```python
from build123d import *

# Parameters (mm, degrees)
CUT_EXTRUDE_1_DEPTH = 2


with BuildPart() as part:
    # 草图1 → 旋转1 (revolve)
    with BuildSketch(Plane.XY):
        with BuildLine():
            Line((0, 10.8), (-2.4, 10.8))
            ThreePointArc((-2.4, 10.8), (-2.682842712, 10.682842712), (-2.8, 10.4))
            Line((-2.8, 10.4), (-2.8, 8.4))
            ThreePointArc((-2.8, 8.4), (-2.682842712, 8.117157288), (-2.4, 8))
            Line((-2.4, 8), (-1.2, 8))
            Line((-1.2, 8), (-1.2, 7))
            Line((-1.2, 7), (-1.5, 7))
            Line((-1.5, 7), (-1.5, 0))
            Line((-1.5, 0), (0, 0))
            Line((0, 0), (0, 10.8))
        make_face()
    revolve(axis=Axis((0, 0, 0), (0, 1, 0)))

    # 草图2 → 切除-拉伸1 (cut)
    with BuildSketch(Plane(origin=(0, 10.8, 0), x_dir=(1, 0, 0), z_dir=(0, 1, 0))):
        Polygon((-0.721687836, 1.25), (-1.443375673, 0), (-0.721687836, -1.25), (0.721687836, -1.25), (1.443375673, 0), (0.721687836, 1.25), align=None)
    extrude(amount=-CUT_EXTRUDE_1_DEPTH, mode=Mode.SUBTRACT)


solid = part.part
```
Verification items for the finished model (mm, model axes). A direction names the side the tool comes from. Coordinates: 2 decimals unless noted, no trailing zeros. Order: outer loops, then holes, each group sorted by start corner. A loop starts at its lowest first (then second) coordinate and runs counter-clockwise, first axis right, second up. Notation, with made-up numbers: (18.25, 13.5) -> (76.25, 13.5) arc R22 cw to (76.25, 47.5) -> close; hole circle Ø1 at (2, -16). An arc over 180 degrees is marked (long way). Put each result on its own line as item: value. Start each with the question number.
1) Tool access check on faces 1 (the cylindrical face through (1.5, 3.45, 0.07)), 2 (the flat face through (-1.088, 9.814, 0.616)), 3 (the flat face through (0, 0, 0)). Record the directions out of +Z, -Z, +X, -X, +Y, -Y that give a thin tool (end or side, any length) a straight path to the whole face; none if there is none.
2) Cross-section at B-B (x = 0). Enter the section's corners in (y, z).
3) Material ranges on L1, parallel to Y at x = -1.7, z = -1.6; L2, parallel to Y at x = -0.75, z = -0.2; L3, parallel to Z at x = 1, y = 9.75, recorded low to high.
4) Cross-section at A-A (y = 9.25). Enter the section's corners in (x, z).
5) Release check for a two-part mould opening along Z. For faces 4 (the flat face through (1.03, 10.8, -1.03)), 5 (the cylindrical face through (-0.65, 7.49, 1.01)), 6 (the flat face through (0, 8.8, 0)) record: pulls with the +Z half, pulls with the -Z half, needs draft (parallel to the pull), parting line crosses it, or undercut.
6) Cross-section at C-C (y = 4). Enter the section's corners in (x, z).
7) Go/stop test with flat-tipped pins: pin 1 (1 mm diameter, centred on y = 1.5, z = 0, fed in from -X); pin 2 (1.5 mm diameter, centred on x = 1.5, y = 8, fed in from +Z); pin 3 (2 mm diameter, centred on x = -1.5, y = 3.5, fed in from +Z). Record where each tip stops, or that it passes through.
Geometry check:
1. face 1: -Y
1. face 2: +Y
1. face 3: +Z, -Z, +X, -X, -Y
2. outline: (0, -1.5) -> (7, -1.5) -> (7, -1.2) -> (8, -1.2) -> (8, -2.4) arc R0.4 ccw to (8.4, -2.8) -> (10.4, -2.8) arc R0.4 ccw to (10.8, -2.4) -> (10.8, -1.25) -> (8.8, -1.25) -> (8.8, 1.25) -> (10.8, 1.25) -> (10.8, 2.4) arc R0.4 ccw to (10.4, 2.8) -> (8.4, 2.8) arc R0.4 ccw to (8, 2.4) -> (8, 1.2) -> (7, 1.2) -> (7, 1.5) -> (0, 1.5) -> close
3. L1: y = 8 to 10.8
3. L2: y = 0 to 8.8
3. L3: z = -2.62 to -0.77, 0.77 to 2.62
4. outline: circle Ø5.6 at (0, 0); hole (-1.44, 0) -> (-0.72, -1.25) -> (0.72, -1.25) -> (1.44, 0) -> (0.72, 1.25) -> (-0.72, 1.25) -> close
5. face 4: needs draft
5. face 5: parting line crosses it
5. face 6: undercut
6. outline: circle Ø3 at (0, 0)
7. pin 1: stops at x = -1.5
7. pin 2: stops at z = 2.67
7. pin 3: stops at z = 1.41
